Check sheet for the drawn part. Datum: minimum x, y, z corner. Units: mm. A direction names the side the tool comes from. Give positions to 0.01 mm unless a question says otherwise; leave off trailing zeros. Loops run counter-clockwise (first coordinate to the right, second up) from the corner with the lowest first, then second, coordinate; pieces in that order, holes last.
1. Release check for a two-part mould opening along X. For the marked faces 3, 4 and 5 record: +X half, -X half, draft (parallel to the pull), parting line (faces both ways), or undercut.
2. Tool access check on the marked faces 1 and 2. Record the directions out of +Z, -Z, +X, -X, +Y, -Y that give a thin tool (end or side, any length) a straight path to the whole face; none if there is none.
3. Material ranges on L1, parallel to Z at x = 18.5, y = 40; L2, parallel to X at y = 43.5, z = 32.5; L3, parallel to Y at x = 7, z = 38, recorded low to high.
4. Cross-section at B-B, the plane x = 41.5. Record the cut outline in (y, z), plus the area to 3 significant figures.
5. Cross-section at A-A, the plane y = 44. Record the cut outline in (x, z).
6. Cross-section at C-C, the plane z = 39. Record the cut outline in (x, y), plus the area to 3 significant figures.
7. Go/stop test with flat-tipped pins: pin 1 Ø12 at (y, z) = (29.5, 20) entering from -X; pin 2 Ø2 at (x, z) = (29.5, 54.5) entering from +Y. Record where each tip stops, or that it passes through.
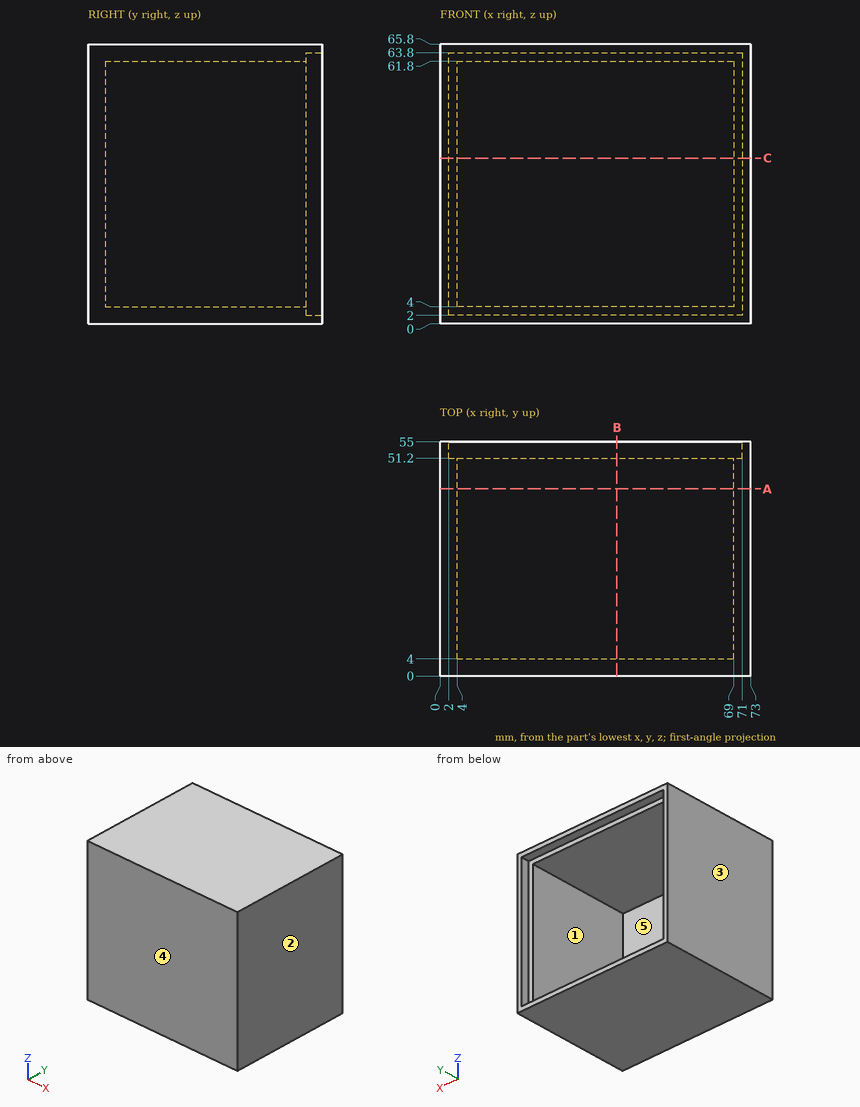
Result:
1. face 3: -X half
1. face 4: draft
1. face 5: undercut
2. face 1: +Y
2. face 2: +Z, -Z, +X, +Y, -Y
3. L1: z = 0 to 4, 61.8 to 65.8
3. L2: x = 0 to 4, 69 to 73
3. L3: y = 0 to 4
4. outline: (0, 0) - (55, 0) - (55, 2) - (51.2, 2) - (51.2, 4) - (4, 4) - (4, 61.8) - (51.2, 61.8) - (51.2, 63.8) - (55, 63.8) - (55, 65.8) - (0, 65.8) - close
4. area: 656 mm2
5. outline: (0, 0) - (73, 0) - (73, 65.8) - (0, 65.8) - close; hole (4, 4) - (69, 4) - (69, 61.8) - (4, 61.8) - close
6. outline: (0, 0) - (73, 0) - (73, 55) - (71, 55) - (71, 51.2) - (69, 51.2) - (69, 4) - (4, 4) - (4, 51.2) - (2, 51.2) - (2, 55) - (0, 55) - close
6. area: 685 mm2
7. pin 1: stops at x = 0
7. pin 2: stops at y = 4
